Source: CAD feature listing. Evaluate the final solid. Frame: model axes, mm. A direction names the side the tool comes from. Give positions to 0.01 mm unless a question says otherwise; leave off trailing zeros. Order: outer loops, then holes, each group sorted by start corner. A loop starts at its lowest first (then second) coordinate and runs counter-clockwise, first axis right, second up. Notation, with made-up numbers: (-26, 52) -> (-15, 52) arc R35 cw to (-15, 86) -> close; hole circle Ø4 at (-39, 20.5). An arc over 180 degrees is marked (long way). Use one line per item in the form item = value. Start each with the question number.
from build123d import *

# Parameters (mm, degrees)
SKETCH2_W             = 17.554431489
SKETCH2_H             = 1.95
BOSS_EXTRUDE1_DEPTH   = 8.75
BOSS_EXTRUDE1_2_DEPTH = 8.75
CUT_EXTRUDE1_DEPTH    = 26.518349076
SKETCH4_W             = 22.027215745
SKETCH4_H             = 12.505427167
BOSS_EXTRUDE2_DEPTH   = 32
SKETCH5_R             = 1.5
CUT_EXTRUDE2_DEPTH    = 12
SKETCH6_W             = 22.027215745
SKETCH6_H             = 12.505427167
SKETCH6_W_2           = 17.554431489
SKETCH6_H_2           = 1.95
CUT_EXTRUDE3_DEPTH    = 2.5
SKETCH7_R             = 1.5
CUT_EXTRUDE4_DEPTH    = 13
SKETCH8_R             = 1.5
CUT_EXTRUDE5_DEPTH    = 28
FILLET3_R             = 1
SKETCH9_W             = 22.02721574
SKETCH9_H             = 2
CUT_EXTRUDE6_DEPTH    = 11


with BuildPart() as part:
    # Sketch2 → Boss-Extrude1 (new body)
    with BuildSketch(Plane.XY):
        with Locations((-13.228930986, -27.845183414)):
            Rectangle(SKETCH2_W, SKETCH2_H)
    extrude(amount=BOSS_EXTRUDE1_DEPTH)


with BuildPart() as body_2:
    # Sketch2 → Boss-Extrude1 2 (new body)
    with BuildSketch(Plane.XY):
        with Locations((-13.228930986, -20.289756247)):
            Rectangle(SKETCH2_W, SKETCH2_H)
    extrude(amount=BOSS_EXTRUDE1_2_DEPTH)


with BuildPart() as cut_extrude1_tool:
    # Sketch3 → Cut-Extrude1 (new, through all)
    with BuildSketch(Plane(origin=(0, -19.314756247, 0), x_dir=(1, 0, 0), z_dir=(0, 1, 0))):
        with BuildLine():
            ThreePointArc((-13.228930986, -8.75), (-7.041746651, -6.187184335), (-4.478930986, 0))
            add(Edge.make_bspline(
                [(-4.478930986, 0), (1.138349918, -4.151657709), (-4.451715242, -8.75)],
                knots=[0, 0, 0, 1, 1, 1], degree=2))
            add(Edge.make_bspline(
                [(-22.006146731, -8.75), (-13.228930986, -12.473510392), (-4.451715242, -8.75)],
                knots=[0, 0, 0, 1, 1, 1], degree=2))
            add(Edge.make_bspline(
                [(-21.978930986, 0), (-25.926969228, -4.242865138), (-22.006146731, -8.75)],
                knots=[0, 0, 0, 1, 1, 1], degree=2))
            ThreePointArc((-21.978930986, 0), (-19.416115322, -6.187184335), (-13.228930986, -8.75))
        make_face()
    extrude(amount=-CUT_EXTRUDE1_DEPTH)


with BuildPart() as part_1:
    add(part.part)

    # Cut-Extrude1: cut by cut_extrude1_tool
    add(cut_extrude1_tool.part, mode=Mode.SUBTRACT)



with BuildPart() as body_2_1:
    add(body_2.part)

    # Cut-Extrude1: cut by cut_extrude1_tool
    add(cut_extrude1_tool.part, mode=Mode.SUBTRACT)


with BuildPart() as part_2:
    add(part_1.part)

    add(body_2_1.part)  # Boss-Extrude2 merges body 2
    # Sketch4 → Boss-Extrude2 (add)
    with BuildSketch(Plane(origin=(0, 0, 0), x_dir=(-1, 0, 0), z_dir=(0, 0, -1))):
        with Locations((13.242538859, -24.067469831)):
            Rectangle(SKETCH4_W, SKETCH4_H)
    extrude(amount=BOSS_EXTRUDE2_DEPTH)

    # Sketch5 → Cut-Extrude2 (cut)
    with BuildSketch(Plane(origin=(0, -19.314756247, 0), x_dir=(1, 0, 0), z_dir=(0, 1, 0))):
        with Locations(Location((-13.228930986, -2.25, 0), (0, 0, 270))):
            Circle(SKETCH5_R)
    extrude(amount=-CUT_EXTRUDE2_DEPTH, mode=Mode.SUBTRACT)

    # Sketch6 → Cut-Extrude3 (cut)
    with BuildSketch(Plane.XY):
        with Locations((-13.242538859, -24.067469831)):
            Rectangle(SKETCH6_W, SKETCH6_H)
        with Locations((-13.228930986, -27.845183414)):
            Rectangle(SKETCH6_W_2, SKETCH6_H_2, mode=Mode.SUBTRACT)
        with Locations((-13.228930986, -20.289756247)):
            Rectangle(SKETCH6_W_2, SKETCH6_H_2, mode=Mode.SUBTRACT)
    extrude(amount=-CUT_EXTRUDE3_DEPTH, mode=Mode.SUBTRACT)

    # Sketch7 → Cut-Extrude4 (cut)
    with BuildSketch(Plane(origin=(0, -17.814756247, 0), x_dir=(1, 0, 0), z_dir=(0, 1, 0))):
        with Locations(Location((-13.242538859, 25.5, 0), (0, 0, 270))):
            Circle(SKETCH7_R)
        with BuildLine():
            Line((-24.086865874, 21.155672985), (-24.256146731, 21.155672985))
            add(Edge.make_bspline(
                [(-2.228930986, 21.155672985), (11.471530889, 27.189710441), (-11.765166974, 53.431279988), (-37.007876173, 21.523583672), (-24.256146731, 21.155672985)],
                knots=[0, 0, 0, 0, 0.52011282, 1, 1, 1, 1], degree=3))
            add(Edge.make_bspline(
                [(-3.948545621, 30.585343246), (-2.007113924, 26.093685314), (-2.228930986, 21.155672985)],
                knots=[0, 0, 0, 1, 1, 1], degree=2))
            Line((-3.948545621, 30.585343246), (-13.242538859, 32))
            ThreePointArc((-13.242538859, 32), (-20.910636028, 28.823770155), (-24.086865874, 21.155672985))
        make_face()
    extrude(amount=-CUT_EXTRUDE4_DEPTH, mode=Mode.SUBTRACT)

    # Sketch8 → Cut-Extrude5 (cut)
    with BuildSketch(Plane.XY.offset(-2.5)):
        with Locations((-18.011106811, -24.06746983)):
            Circle(SKETCH8_R)
        with Locations((-8.473970906, -24.06746983)):
            Circle(SKETCH8_R)
    extrude(amount=-CUT_EXTRUDE5_DEPTH, mode=Mode.SUBTRACT)

    # Fillet3
    # the kernel refuses this fillet: 1 mm, written as the material it takes off along each edge
    with BuildSketch(Plane(origin=(-24.256146731, -15.314756247, -2.5), x_dir=(1, 0, 0), z_dir=(0, -1, 0))) as fillet3_piece_1:
        with BuildLine():
            CenterArc((FILLET3_R, -FILLET3_R), FILLET3_R, 90, 90)
            Line((0, -FILLET3_R), (-FILLET3_R * 0.02, -FILLET3_R))
            Line((-FILLET3_R * 0.02, -FILLET3_R), (-FILLET3_R * 0.02, FILLET3_R * 0.02))
            Line((-FILLET3_R * 0.02, FILLET3_R * 0.02), (FILLET3_R, FILLET3_R * 0.02))
            Line((FILLET3_R, FILLET3_R * 0.02), (FILLET3_R, 0))
        make_face()
    extrude(amount=17.505427167, mode=Mode.SUBTRACT)
    with BuildSketch(Plane(origin=(-24.256146731, -16.423026869, -21.155672985), x_dir=(0, 0, 1), z_dir=(0, -1, 0))) as fillet3_piece_2:
        with BuildLine():
            CenterArc((0.556691751, -1), FILLET3_R, 90, 33.827317624)
            Line((0, -0.169280857), (-0.011133835, -0.152666474))
            ThreePointArc((-0.011133835, -0.152666474), (-0.02, -0.084640429), (-0.02, 0))
            Line((-0.02, 0), (0, 0.02))
            Line((0, 0.02), (0.556691751, 0.02))
            Line((0.556691751, 0.02), (0.556691751, 0))
        make_face()
    extrude(amount=15.288885922, mode=Mode.SUBTRACT)
    with BuildSketch(Plane(origin=(-2.228930986, -32.820183414, -2.5), x_dir=(0, 0, -1), z_dir=(0, 1, 0))) as fillet3_piece_3:
        with BuildLine():
            CenterArc((FILLET3_R, FILLET3_R), FILLET3_R, 180, 90)
            Line((0, FILLET3_R), (-FILLET3_R * 0.02, FILLET3_R))
            Line((-FILLET3_R * 0.02, FILLET3_R), (-FILLET3_R * 0.02, -FILLET3_R * 0.02))
            Line((-FILLET3_R * 0.02, -FILLET3_R * 0.02), (FILLET3_R, -FILLET3_R * 0.02))
            Line((FILLET3_R, -FILLET3_R * 0.02), (FILLET3_R, 0))
        make_face()
    extrude(amount=17.505427167, mode=Mode.SUBTRACT)
    with BuildSketch(Plane(origin=(-3.948545621, -16.375444783, -30.585343246), x_dir=(-0.9886132451058307, 0, -0.1504787413600958), z_dir=(0, -1, 0))) as fillet3_piece_4:
        with BuildLine():
            CenterArc((0.562435527, -1), FILLET3_R, 90, 59.471323616)
            Line((-0.298939504, -0.492030458), (-0.316167005, -0.481871067))
            ThreePointArc((-0.316167005, -0.481871067), (-0.168173949, -0.234650824), (-0.016955383, 0.010607308))
            Line((-0.016955383, 0.010607308), (0, 0.02))
            Line((0, 0.02), (0.562435527, 0.02))
            Line((0.562435527, 0.02), (0.562435527, 0))
        make_face()
    extrude(amount=15.384050094, mode=Mode.SUBTRACT)

    # Sketch9 → Cut-Extrude6 (cut)
    with BuildSketch(Plane.XY.offset(-32.5)):
        with Locations((-13.24253886, -20.31475625)):
            Rectangle(SKETCH9_W, SKETCH9_H)
        with Locations((-13.24253886, -27.836055834)):
            Rectangle(SKETCH9_W, SKETCH9_H)
    extrude(amount=CUT_EXTRUDE6_DEPTH, mode=Mode.SUBTRACT)


solid = part_2.part
1) Draft query along X for faces 6 (the face through (-4.452, -20, -1)), 7 (the face through (-15, -21.265, 2)), 8 (the face through (-14.693, -27.832, 1.925)). Return one class per face: +X half, -X half, draft (parallel to the pull), parting line (faces both ways), or undercut.
2) Cut plane D-D, the plane x = -9.5. Return the cut outline in (y, z).
3) Cut plane B-B, the plane z = -7.5. Return the cut outline in (x, y), plus the area to 3 significant figures.
4) Reachability of faces 1 (the face through (-22.006, -20, -1)), 2 (the face through (-15, -28.82, 2)), 3 (the face through (-15, -19.315, 2)), 4 (the face through (-19.51, -24, -16.3)), 5 (the face through (-13, -20, -21.5)) from +Z, -Z, +X, -X, +Y, -Y: full face, straight path, thin tool, end or side. Return the list, or none.
5) Cut plane C-C, the plane z = -27.5. Count the separate pieces of the cut face and the enclosed holes in it, plus the area to 3 significant figures.
6) Pin query (flat end, axial travel): pin 1 (1.5 mm diameter, centred on x = -15, y = -27.5, fed in from +Z); pin 2 (12.5 mm diameter, centred on x = -17, z = 3, fed in from -Y); pin 3 (1 mm diameter, centred on x = -8, y = -20, fed in from -Z); pin 4 (1.6 mm diameter, centred on x = -9.5, y = -27.5, fed in from -Z). Return the tip coordinate at first contact, or that it passes through.
7) Cut plane A-A, the plane z = 2.25. Return the cut outline in (x, y), plus the area to 3 significant figures.
8) Material intervals for probe 1 along Y at (x, z) = (-22.5, -25); probe 2 along Y at (x, z) = (-8, 1); probe 3 along Y at (x, z) = (-9.5, -29), sorted ascending.
Output values:
q1.face_6 = +X half
q1.face_7 = draft
q1.face_8 = undercut
q2.outline = (-30.32, -31.43) -> (-28.84, -31.43) -> (-28.84, -21.5) -> (-26.84, -21.5) -> (-26.84, -31.43) -> (-21.31, -31.43) -> (-21.31, -21.5) -> (-19.31, -21.5) -> (-19.31, -31.43) -> (-17.81, -31.43) -> (-17.81, -2.5) -> (-19.31, -2.5) -> (-19.31, 7.92) -> (-21.26, 7.92) -> (-21.26, -2.5) -> (-22.97, -2.5) -> (-22.97, -30.5) -> (-25.16, -30.5) -> (-25.16, -2.5) -> (-26.87, -2.5) -> (-26.87, 7.92) -> (-28.82, 7.92) -> (-28.82, -2.5) -> (-30.32, -2.5) -> close
q3.outline = (-24.26, -30.32) -> (-2.23, -30.32) -> (-2.23, -17.81) -> (-24.26, -17.81) -> close; hole circle Ø3 at (-18.01, -24.07); hole circle Ø3 at (-8.47, -24.07)
q3.area = 261 mm^2
q4.face_1 = +Z, -X, +Y, -Y
q4.face_2 = +Z, +X, -X, -Y
q4.face_3 = +Z, +X, -X, +Y
q4.face_4 = +Z
q4.face_5 = -Z, +X, -X
q5.separate_pieces = 3
q5.enclosed_holes = 2
q5.area = 149 mm^2
q6.pin_1 = 8.69
q6.pin_2 = -30.32
q6.pin_3 = -21.5
q6.pin_4 = -31.5
q7.outline = (-21.68, -28.82) -> (-14.73, -28.82) -> (-14.73, -26.87) -> (-21.68, -26.87) -> close; (-21.68, -21.26) -> (-14.73, -21.26) -> (-14.73, -19.31) -> (-21.68, -19.31) -> close; (-11.73, -28.82) -> (-4.77, -28.82) -> (-4.77, -26.87) -> (-11.73, -26.87) -> close; (-11.73, -21.26) -> (-4.77, -21.26) -> (-4.77, -19.31) -> (-11.73, -19.31) -> close
q7.area = 54.3 mm^2
q8.probe_1 = -30.32 to -28.84, -26.84 to -21.31, -19.31 to -17.81
q8.probe_2 = -28.82 to -26.87, -21.26 to -19.31
q8.probe_3 = -30.32 to -28.84, -26.84 to -25.16, -22.97 to -21.31, -19.31 to -17.81
